```python
from build123d import *

# Parameters (mm, degrees)
F0_W         = 25.4
F0_H         = 50.8
F0_W_2       = 6.35
F1_DEPTH     = 6.35
F2_DEPTH     = 12.7
F3_R         = 3.17499
F4_T1_DEPTH  = 30.16251
F4_T3_DEPTH  = 44.45001
F4_T5_DEPTH  = 17.46251
F4_T7_DEPTH  = 3.17501
F4_T10_ANGLE = 90
F4_T12_ANGLE = 90
F4_T14_ANGLE = 90
F4_T16_ANGLE = 90
F4_T18_ANGLE = 90
F4_T20_ANGLE = 90
F4_T22_ANGLE = 90
F4_T24_ANGLE = 90


# Not quite as in the source:
# - a fillet or chamfer that OpenCascade refuses, or shapes differently, is made with other operations: its cross-section is extruded or revolved along the edge and cut away or added
# - a fillet or chamfer is up to 0.001 mm smaller than in the source, because OpenCascade refuses the exact size


with BuildPart() as f1:
    # F0 (on Front) → F1 (new body)
    with BuildSketch(Plane.XZ):
        with Locations((-19.05, 25.4)):
            Rectangle(F0_W, F0_H)
        with Locations((-3.175, 25.4)):
            Rectangle(F0_W_2, F0_H)
    extrude(amount=F1_DEPTH)

    # F0 (on Front) → F2 (join)
    with BuildSketch(Plane.XZ):
        with Locations((-3.175, 25.4)):
            Rectangle(F0_W_2, F0_H)
    extrude(amount=F2_DEPTH)

    # F3 (radius 3.175 in the source; OpenCascade refuses exactly that, so slightly less here)
    f3_edges = [f1.edges().sort_by_distance(p)[0] for p in [
        (0, 0, 25.4),
        (-6.35, -6.35, 25.4),
        (-3.175, -12.7, 0),
        (0, -12.7, 25.4),
        (-3.175, -12.7, 50.8),
        (-6.35, -12.7, 25.4),
    ]]
    fillet(f3_edges, radius=F3_R)

    # F4: fillet of radius 3.175 on 4 edges, made by hand

    # F4_s2 → F4_t1 (cut)
    with BuildSketch(Plane.YZ.offset(-39.6875)):
        with BuildLine():
            ThreePointArc((-6.35, 47.625), (-5.4200640303, 49.8700640303), (-3.175, 50.8))
            Line((-3.175, 50.8), (-6.35, 50.8))
            Line((-6.35, 50.8), (-6.35, 47.625))
        make_face()
        with BuildLine():
            ThreePointArc((-6.35, 3.175), (-5.4200640303, 0.9299359697), (-3.175, 0))
            Line((-3.175, 0), (-6.35, 0))
            Line((-6.35, 0), (-6.35, 3.175))
        make_face()
    extrude(amount=F4_T1_DEPTH, mode=Mode.SUBTRACT)

    # F4_s4 → F4_t3 (cut)
    with BuildSketch(Plane.YZ.offset(-39.6875)):
        with BuildLine():
            ThreePointArc((-3.175, 0), (-0.9299359697, 0.9299359697), (0, 3.175))
            Line((0, 3.175), (0, 0))
            Line((0, 0), (-3.175, 0))
        make_face()
        with BuildLine():
            ThreePointArc((-3.175, 50.8), (-0.9299359697, 49.8700640303), (0, 47.625))
            Line((0, 47.625), (0, 50.8))
            Line((0, 50.8), (-3.175, 50.8))
        make_face()
    extrude(amount=F4_T3_DEPTH, mode=Mode.SUBTRACT)

    # F4_s6 → F4_t5 (cut)
    with BuildSketch(Plane.XZ.offset(-4.76251)):
        with BuildLine():
            ThreePointArc((-3.175, 50.8), (-0.9299359697, 49.8700640303), (0, 47.625))
            Line((0, 47.625), (0, 50.8))
            Line((0, 50.8), (-3.175, 50.8))
        make_face()
        with BuildLine():
            ThreePointArc((-3.175, 0), (-0.9299359697, 0.9299359697), (0, 3.175))
            Line((0, 3.175), (0, 0))
            Line((0, 0), (-3.175, 0))
        make_face()
    extrude(amount=F4_T5_DEPTH, mode=Mode.SUBTRACT)

    # F4_s8 → F4_t7 (cut)
    with BuildSketch(Plane.XZ.offset(9.52499)):
        with BuildLine():
            ThreePointArc((-3.175, 0), (-5.4200640303, 0.9299359697), (-6.35, 3.175))
            Line((-6.35, 3.175), (-6.35, 0))
            Line((-6.35, 0), (-3.175, 0))
        make_face()
        with BuildLine():
            ThreePointArc((-3.175, 50.8), (-5.4200640303, 49.8700640303), (-6.35, 47.625))
            Line((-6.35, 47.625), (-6.35, 50.8))
            Line((-6.35, 50.8), (-3.175, 50.8))
        make_face()
    extrude(amount=F4_T7_DEPTH, mode=Mode.SUBTRACT)

    # F4_s9 → F4_t10 (revolve, cut)
    with BuildSketch(Plane.XY.offset(47.625)):
        with BuildLine():
            ThreePointArc((-3.17499, -12.7), (-0.9299330408, -11.7700669592), (0, -9.52501))
            Line((0, -9.52501), (0, -12.7))
            Line((0, -12.7), (-3.17499, -12.7))
        make_face()
    revolve(axis=Axis((-3.175, -12.7, 47.625), (0, -1, 0)), revolution_arc=F4_T10_ANGLE, mode=Mode.SUBTRACT)

    # F4_s11 → F4_t12 (revolve, cut)
    with BuildSketch(Plane.YZ.offset(-3.175)):
        with BuildLine():
            ThreePointArc((-12.7, 3.17499), (-11.7700669592, 0.9299330408), (-9.52501, 0))
            Line((-9.52501, 0), (-12.7, 0))
            Line((-12.7, 0), (-12.7, 3.17499))
        make_face()
    revolve(axis=Axis((-3.175, -12.7, 3.175), (0, -1, 0)), revolution_arc=F4_T12_ANGLE, mode=Mode.SUBTRACT)

    # F4_s13 → F4_t14 (revolve, cut)
    with BuildSketch(Plane.XY.offset(3.175)):
        with BuildLine():
            ThreePointArc((-3.17501, -12.7), (-5.4200669592, -11.7700669592), (-6.35, -9.52501))
            Line((-6.35, -9.52501), (-6.35, -12.7))
            Line((-6.35, -12.7), (-3.17501, -12.7))
        make_face()
    revolve(axis=Axis((-3.175, -12.7, 3.175), (0, -1, 0)), revolution_arc=F4_T14_ANGLE, mode=Mode.SUBTRACT)

    # F4_s15 → F4_t16 (revolve, cut)
    with BuildSketch(Plane.YZ.offset(-3.175)):
        with BuildLine():
            ThreePointArc((-12.7, 47.62501), (-11.7700669592, 49.8700669592), (-9.52501, 50.8))
            Line((-9.52501, 50.8), (-12.7, 50.8))
            Line((-12.7, 50.8), (-12.7, 47.62501))
        make_face()
    revolve(axis=Axis((-3.175, -12.7, 47.625), (0, -1, 0)), revolution_arc=F4_T16_ANGLE, mode=Mode.SUBTRACT)

    # F4_s17 → F4_t18 (revolve, cut)
    with BuildSketch(Plane.XZ.offset(3.17499)):
        with BuildLine():
            ThreePointArc((-3.17499, 50.8), (-0.9299324342, 49.8700604947), (0, 47.625))
            Line((0, 47.625), (0, 50.8))
            Line((0, 50.8), (-3.17499, 50.8))
        make_face()
    revolve(axis=Axis((-3.17499, -3.17499, 50.8), (0, 0, 1)), revolution_arc=F4_T18_ANGLE, mode=Mode.SUBTRACT)

    # F4_s19 → F4_t20 (revolve, cut)
    with BuildSketch(Plane.XZ.offset(3.17499)):
        with BuildLine():
            ThreePointArc((-3.17499, 0), (-0.9299324342, 0.9299395053), (0, 3.175))
            Line((0, 3.175), (0, 0))
            Line((0, 0), (-3.17499, 0))
        make_face()
    revolve(axis=Axis((-3.17499, -3.17499, 0), (0, 0, 1)), revolution_arc=F4_T20_ANGLE, mode=Mode.SUBTRACT)

    # F4_s21 → F4_t22 (revolve, cut)
    with BuildSketch(Plane.YZ.offset(-9.52499)):
        with BuildLine():
            ThreePointArc((-6.35, 3.175), (-5.4200640303, 0.9299359697), (-3.175, 0))
            Line((-3.175, 0), (-6.35, 0))
            Line((-6.35, 0), (-6.35, 3.175))
        make_face()
    revolve(axis=Axis((-9.52499, -9.52499, 0), (0, 0, -1)), revolution_arc=F4_T22_ANGLE, mode=Mode.SUBTRACT)

    # F4_s23 → F4_t24 (revolve, cut)
    with BuildSketch(Plane.YZ.offset(-9.52499)):
        with BuildLine():
            ThreePointArc((-3.175, 50.8), (-5.4200640303, 49.8700640303), (-6.35, 47.625))
            Line((-6.35, 47.625), (-6.35, 50.8))
            Line((-6.35, 50.8), (-3.175, 50.8))
        make_face()
    revolve(axis=Axis((-9.52499, -9.52499, 50.8), (0, 0, -1)), revolution_arc=F4_T24_ANGLE, mode=Mode.SUBTRACT)


solid = f1.part
```
For this review, take the finished solid that the model builds, in its own axes (mm). A direction names the side the tool comes from. Give positions to 0.01 mm unless a question says otherwise; leave off trailing zeros. Write each loop counter-clockwise with the first axis right and the second up, starting at its lowest first coordinate (ties: lowest second). Pieces come first, ordered by that corner, then holes.
Item 1: Take a section at B-B (x = -14.5). Give the boundary of the cut face in (y, z) (3 decimals), and give its area (3 significant figures).
Item 2: Machinability: for faces 1 (the face through (-5, -4, 0)), 2 (the face through (-21, -6.35, 26)), which of the approach directions +Z, -Z, +X, -X, +Y, -Y give a long, thin tool a straight path to every point of the face, cutting with its end or side? Answer none if there is none.
Item 3: Insertion check: P1, Ø3, axis at x = -27.5, z = 13, coming from the -Y side; P2, Ø1, axis at y = -11.5, z = 13.5, coming from the +X side; P3, Ø12, axis at x = -4.5, z = 6.5, coming from the -Y side. Each pin has a flat end and moves straight along its axis. Give the tip position at first contact, or say it passes through.
Item 4: Wall thickness on probe 1 along Z at (x, y) = (-19.5, -3); probe 2 along Y at (x, z) = (-14, 19): over which ranges is each line inside the solid? List them lowest first.
Established:
1. outline: (-6.35, 3.175) arc R3.175 ccw to (0, 3.175) - (0, 47.625) arc R3.175 ccw to (-6.35, 47.625) - close
1. area: 314 mm2
2. face 1: -Z, +X, -X, +Y, -Y
2. face 2: +Z, -Z, -X, -Y
3. P1: stops at y = -6.35
3. P2: stops at x = -0.36
3. P3: stops at y = -12.7
4. probe 1: z = 0 to 50.8
4. probe 2: y = -6.35 to 0
